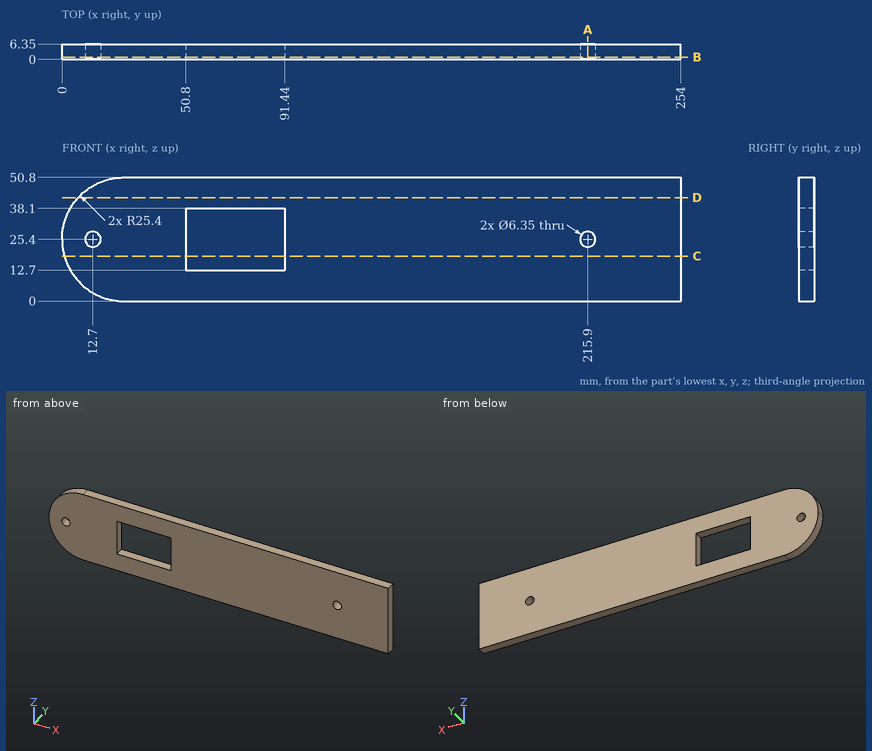
Input: dimensioned drawing with shaded views. Units: mm. Origin: part minimum x, y, z. Give positions to 0.01 mm unless a question says otherwise; leave off trailing zeros. Loops run counter-clockwise (first coordinate to the right, second up) from the corner with the lowest first, then second, coordinate; pieces in that order, holes last. Notation, with made-up numbers: (77.25, 42) -> (128.25, 42) arc R14 ccw to (128.25, 47) -> close; hole circle Ø10 at (89.25, -32.75). An arc over 180 degrees is marked (long way). Return JSON: item names as keys, results as strings.
Item 1: Pin query (flat end, axial travel): P1, Ø2, axis at y = 2.5, z = 36, coming from the -X side; P2, Ø1.9, axis at y = 3, z = 28.5, coming from the -X side. Return the tip coordinate at first contact, or that it passes through.
Filled in:
{"P1": "x = 1.88", "P2": "x = 0.09"}
Item 2: Section C-C, the plane z = 18.5. Output: boundary loops of the cut face in (x, y) (3 decimals).
Filled in:
{"outline": "(0.955, 0) -> (50.8, 0) -> (50.8, 6.35) -> (0.955, 6.35) -> close; (91.44, 0) -> (254, 0) -> (254, 6.35) -> (91.44, 6.35) -> close"}
Item 3: Section D-D, the plane z = 42.5. Output: boundary loops of the cut face in (x, y), plus the area to 3 significant figures.
Filled in:
{"outline": "(6.62, 0) -> (254, 0) -> (254, 6.35) -> (6.62, 6.35) -> close", "area": "1,570 mm^2"}
Item 4: Line query: line 1 (Z direction, x = 215.9, y = 4) (3 decimals); line 2 (X direction, y = 1, z = 22.5) (1 decimal); line 3 (Z direction, x = 68.5, y = 4.5). Output: solid intervals per line, ascending.
Filled in:
{"line 1": "0 to 22.225, 28.575 to 50.8", "line 2": "0.2 to 11.4, 14 to 50.8, 91.4 to 214.6, 217.2 to 254", "line 3": "0 to 12.7, 38.1 to 50.8"}
Item 5: Section A-A, the plane x = 215.9. Output: boundary loops of the cut face in (y, z) (3 decimals), plus the area to 3 significant figures.
Filled in:
{"outline": "(0, 0) -> (6.35, 0) -> (6.35, 22.225) -> (0, 22.225) -> close; (0, 28.575) -> (6.35, 28.575) -> (6.35, 50.8) -> (0, 50.8) -> close", "area": "282 mm^2"}
Item 6: Section B-B, the plane y = 1. Count the separate pieces of the cut face and the enclosed holes in it, plus the area to 3 significant figures.
Filled in:
{"separate pieces": "1", "enclosed holes": "3", "area": "11,500 mm^2"}
